```python
from build123d import *

# Parameters (mm, degrees)
SKETCH1_R           = 50
BOSS_EXTRUDE2_DEPTH = 15
SHELL1_T            = -4
SKETCH3_R           = 27.405
BOSS_EXTRUDE3_DEPTH = 4
SKETCH7_R           = 2.5
CUT_EXTRUDE1_DEPTH  = 12
BOSS_EXTRUDE5_START = 12
SKETCH8_R           = 50
SKETCH8_R_2         = 48
BOSS_EXTRUDE5_DEPTH = 12


with BuildPart() as part:
    # Sketch1 → Boss-Extrude2 (new body)
    with BuildSketch(Plane(origin=(0, 0, 0), x_dir=(1, 0, 0), z_dir=(0, 1, 0))):
        with Locations(Location((0, 0, 0), (0, 0, 270))):
            Circle(SKETCH1_R)
    extrude(amount=BOSS_EXTRUDE2_DEPTH)

    # Shell1
    shell1_openings = [part.faces().sort_by_distance(p)[0] for p in [
        (0, 15, 0),
    ]]
    offset(amount=SHELL1_T, openings=shell1_openings, kind=Kind.INTERSECTION)

    # Sketch3 → Boss-Extrude3 (add)
    with BuildSketch(Plane(origin=(0, 4, 0), x_dir=(1, 0, 0), z_dir=(0, 1, 0))):
        with Locations(Location((0, 0, 0), (0, 0, 270))):
            Circle(SKETCH3_R)
    extrude(amount=BOSS_EXTRUDE3_DEPTH)

    # Sketch7 → Cut-Extrude1 (cut)
    with BuildSketch(Plane(origin=(0, 8, 0), x_dir=(1, 0, 0), z_dir=(0, 1, 0))):
        with Locations(Location((35, 0, 0), (0, 0, 270))):
            Circle(SKETCH7_R)
        with Locations(Location((0, 35, 0), (0, 0, 270))):
            Circle(SKETCH7_R)
        with Locations(Location((-35, 0, 0), (0, 0, 270))):
            Circle(SKETCH7_R)
        with Locations(Location((0, -35, 0), (0, 0, 270))):
            Circle(SKETCH7_R)
    extrude(amount=-CUT_EXTRUDE1_DEPTH, mode=Mode.SUBTRACT)

    # Sketch8 → Boss-Extrude5 (add)
    with BuildSketch(Plane(origin=(0, 0, 0), x_dir=(-1, 0, 0), z_dir=(0, -1, 0)).offset(BOSS_EXTRUDE5_START)):
        with Locations(Location((0, 0, 0), (0, 0, 90))):
            Circle(SKETCH8_R)
        with Locations(Location((0, 0, 0), (0, 0, 90))):
            Circle(SKETCH8_R_2, mode=Mode.SUBTRACT)
    extrude(amount=-BOSS_EXTRUDE5_DEPTH)


solid = part.part
```
Design review of the part built by this model. Coordinates are the model's own, in mm. A direction names the side the tool comes from. Coordinates: 2 decimals unless noted, no trailing zeros. Order: outer loops, then holes, each group sorted by start corner. A loop starts at its lowest first (then second) coordinate and runs counter-clockwise, first axis right, second up.
1) Take a section at B-B, the plane x = 0. Give the boundary of the cut face in (y, z) (3 decimals).
2) Take a section at A-A, the plane z = 0. Give the boundary of the cut face in (x, y) (3 decimals), and give its area (3 significant figures).
3) Take a section at D-D, the plane z = -35. Give the boundary of the cut face in (x, y), and give its area (3 significant figures).
4) For faces 1 (the flat face through (1, 0, -1)), 2 (the cylindrical face through (-0.96, 2.03, 37.31)), 3 (the flat face through (0, 8, 0)), list the 3-axis set-ups (+Z, -Z, +X, -X, +Y, -Y) from which the entire face can be reached by the end or side of a thin tool; tool diameter is ignored.
5) Clearance check with flat-ended pins moving along their axes: pin 1 (5 mm diameter, centred on x = 1.5, z = -4, fed in from +Y); pin 2 (4 mm diameter, centred on x = -38, z = 21.5, fed in from -Y); pin 3 (6.5 mm diameter, centred on x = 35, z = 0, fed in from +Y). State where each tip first meets the part, or that it passes through.
6) Take a section at C-C, the plane y = 2.5. Give the boundary of the cut face in (x, z).
7) Mouldability with a two-part tool opening along Z and no side actions: class faces 4 (the flat face through (19, -12, 45)), 5 (the cylindrical face through (32.56, 2.03, -0.54)) as +Z half, -Z half, draft (parallel to the pull), parting line (faces both ways), or undercut.
8) Wall thickness on line 1 along X through (y, z) = (1.55, 0); line 2 along Z through (x, y) = (0, 9); line 3 along Y through (x, z) = (32, -5): over which ranges is each line inside the solid? List them lowest first.
Returned:
1. outline: (-12, -50) - (15, -50) - (15, -46) - (4, -46) - (4, -37.5) - (0, -37.5) - (0, -48) - (-12, -48) - close; (-12, 48) - (0, 48) - (0, 37.5) - (4, 37.5) - (4, 46) - (15, 46) - (15, 50) - (-12, 50) - close; (0, -32.5) - (4, -32.5) - (4, -27.405) - (8, -27.405) - (8, 27.405) - (4, 27.405) - (4, 32.5) - (0, 32.5) - close
2. outline: (-50, -12) - (-48, -12) - (-48, 0) - (-37.5, 0) - (-37.5, 4) - (-46, 4) - (-46, 15) - (-50, 15) - close; (-32.5, 0) - (32.5, 0) - (32.5, 4) - (27.405, 4) - (27.405, 8) - (-27.405, 8) - (-27.405, 4) - (-32.5, 4) - close; (37.5, 0) - (48, 0) - (48, -12) - (50, -12) - (50, 15) - (46, 15) - (46, 4) - (37.5, 4) - close
2. area: 715 mm2
3. outline: (-35.71, -12) - (-32.85, -12) - (-32.85, 0) - (-2.5, 0) - (-2.5, 4) - (-29.85, 4) - (-29.85, 15) - (-35.71, 15) - close; (2.5, 0) - (32.85, 0) - (32.85, -12) - (35.71, -12) - (35.71, 15) - (29.85, 15) - (29.85, 4) - (2.5, 4) - close
3. area: 463 mm2
4. face 1: -Y
4. face 2: +Y, -Y
4. face 3: +Y
5. pin 1: stops at y = 8
5. pin 2: stops at y = 0
5. pin 3: stops at y = 4
6. outline: circle Ø100 at (0, 0); hole circle Ø5 at (-35, 0); hole circle Ø5 at (0, -35); hole circle Ø5 at (0, 35); hole circle Ø5 at (35, 0)
7. face 4: draft
7. face 5: undercut
8. line 1: x = -50 to -37.5, -32.5 to 32.5, 37.5 to 50
8. line 2: z = -50 to -46, 46 to 50
8. line 3: y = 0 to 4
